```python
from build123d import *

# Parameters (mm, degrees)
REFERENCE_R            = 6.35
REFERENCE_R_2          = 3.175
REFERENCE_R_3          = 4.2545
BOSS_EXTRUDE3_DEPTH    = 6.604
F_10_32_TAPPED_HOLE1_D = 4.0386
SKETCH3_R              = 2.5796875
CUT_EXTRUDE1_DEPTH     = 369.153899125
SKETCH4_R              = 2.5796875
CUT_EXTRUDE2_DEPTH     = 369.153899125
SKETCH5_R              = 4.7625
CUT_EXTRUDE3_DEPTH     = 369.153899125


with BuildPart() as part:
    # reference → Boss-Extrude3 (new body)
    with BuildSketch(Plane.XY):
        Polygon((206.375, 0), (-206.375, 0), (-206.375, 171.45), (-72.7075, 304.8), (72.7075, 304.8), (206.375, 171.45), align=None)
        with Locations(Location((-100.0125, 112.7125, 0), (0, 0, 180))):
            Circle(REFERENCE_R, mode=Mode.SUBTRACT)
        with Locations(Location((100.0125, 112.7125, 0), (0, 0, 180))):
            Circle(REFERENCE_R, mode=Mode.SUBTRACT)
        with Locations(Location((-66.675, 254, 0), (0, 0, 180))):
            Circle(REFERENCE_R_2, mode=Mode.SUBTRACT)
        with Locations(Location((58.42, 254, 0), (0, 0, 180))):
            Circle(REFERENCE_R_3, mode=Mode.SUBTRACT)
    extrude(amount=BOSS_EXTRUDE3_DEPTH)

    # #10-32 Tapped Hole1 (through all)
    with Locations(Plane.XY.offset(6.604)):
        with Locations((-167.64, 26.9875), (167.64, 27.0002), (-28.575, 284.734), (22.225, 284.734), (-28.575, 254), (22.225, 254)):
            Hole(F_10_32_TAPPED_HOLE1_D / 2)

    # Sketch3 → Cut-Extrude1 (cut, through all)
    with BuildSketch(Plane(origin=(0, 0, 0), x_dir=(-1, 0, 0), z_dir=(0, 0, -1))):
        with Locations((-33.62112915, 278.748737342)):
            Circle(SKETCH3_R)
        with Locations((-33.62112915, 229.251262658)):
            Circle(SKETCH3_R)
        with Locations((-83.118603833, 229.251262658)):
            Circle(SKETCH3_R)
        with Locations((-83.118603833, 278.748737342)):
            Circle(SKETCH3_R)
    extrude(amount=-CUT_EXTRUDE1_DEPTH, mode=Mode.SUBTRACT)

    # Sketch4 → Cut-Extrude2 (cut, through all)
    with BuildSketch(Plane.XY.offset(6.604)):
        with Locations((-28.575, 215.9)):
            Circle(SKETCH4_R)
        with Locations((22.225, 215.9)):
            Circle(SKETCH4_R)
        with Locations((-15.875, 180.594)):
            Circle(SKETCH4_R)
        with Locations((9.525, 180.594)):
            Circle(SKETCH4_R)
    extrude(amount=-CUT_EXTRUDE2_DEPTH, mode=Mode.SUBTRACT)

    # Sketch5 → Cut-Extrude3 (cut, through all)
    with BuildSketch(Plane(origin=(0, 0, 0), x_dir=(-1, 0, 0), z_dir=(0, 0, -1))):
        with Locations((-193.675, 166.18063958)):
            Circle(SKETCH5_R)
        with Locations(Location((193.675, 166.18063958, 0), (0, 0, 180))):
            Circle(SKETCH5_R)
    extrude(amount=-CUT_EXTRUDE3_DEPTH, mode=Mode.SUBTRACT)


solid = part.part
```
Source: CAD feature listing. Evaluate the final solid. Frame: model axes, mm. Coordinates: 2 decimals unless noted, no trailing zeros. Write each loop counter-clockwise with the first axis right and the second up, starting at its lowest first coordinate (ties: lowest second). Pieces come first, ordered by that corner, then holes. Notation, with made-up numbers: (-28.5, 85.25) - (0.5, 85.25) arc R25 ccw to (0.5, 101.25) - close; hole circle Ø1 at (-17, 24). An arc over 180 degrees is marked (long way). Answer as a JSON object with one key per item and string values.
Q1. Material intervals for line 1 (X direction, y = 170, z = 6) (3 decimals); line 2 (X direction, y = 256.5, z = 6.5); line 3 (X direction, y = 254.5, z = 3.5), sorted ascending. Write a range as [from, to].
Ans:
{"line 1": "x = [-206.375, -196.52], [-190.83, 190.83], [196.52, 206.375]", "line 2": "x = [-121.12, -68.63], [-64.72, 54.98], [61.86, 121.12]", "line 3": "x = [-123.13, -69.81], [-63.54, -30.53], [-26.62, 20.27], [24.18, 54.19], [62.65, 123.13]"}
Q2. Section query A-A, the plane x = 58.42. Output: boundary loops of the cut face in (y, z), plus the area to 3 significant figures.
Ans:
{"outline": "(0, 0) - (249.75, 0) - (249.75, 6.6) - (0, 6.6) - close; (258.25, 0) - (304.8, 0) - (304.8, 6.6) - (258.25, 6.6) - close", "area": "1,960 mm2"}
Q3. Section query C-C, the plane x = 102. Output: boundary loops of the cut face in (y, z), plus the area to 3 significant figures.
Ans:
{"outline": "(0, 0) - (106.68, 0) - (106.68, 6.6) - (0, 6.6) - close; (118.74, 0) - (275.58, 0) - (275.58, 6.6) - (118.74, 6.6) - close", "area": "1,740 mm2"}
Q4. Draft query along Y for faces 1 (the flat face through (3, 121, 6.604)), 2 (the cylindrical face through (58.97, 249.78, 3.26)), 3 (the flat face through (-140.48, 237.19, 3.26)). Return one class per face: released by +Y, released by -Y, zero draft, split by the parting line, or undercut.
Ans:
{"face 1": "zero draft", "face 2": "undercut", "face 3": "released by +Y"}
Q5. Section query B-B, the plane z = 3.5. State how many separate pieces and enclosed holes the cut face has, plus the area to 3 significant figures.
Ans:
{"separate pieces": "1", "enclosed holes": "20", "area": "107,000 mm2"}
Q6. First-contact query: pin 1 Ø4.5 at (x, y) = (33.62, 278.75) entering from +Z; pin 2 Ø11 at (x, y) = (58.42, 254) entering from +Z; pin 3 Ø3 at (x, z) = (84.5, 1) entering from +Y. Flat tips, straight axial feed; report the tip coordinate or a pass-through.
Ans:
{"pin 1": "passes through", "pin 2": "stops at z = 6.6", "pin 3": "stops at y = 294.53"}
